Input: part model. Units: mm. Frame: model coordinates. Face numbers are marked on the shaded views. A direction names the side the tool comes from. Give positions to 0.01 mm unless a question says otherwise; leave off trailing zeros. Loops run counter-clockwise (first coordinate to the right, second up) from the corner with the lowest first, then second, coordinate; pieces in that order, holes last. Notation, with made-up numbers: (-1, 73) -> (3, 73) arc R12 cw to (3, 88) -> close; hole circle Ø6 at (30.5, 68). An arc over 180 degrees is marked (long way). Answer in a Markdown table with one row per item. Add a question column.
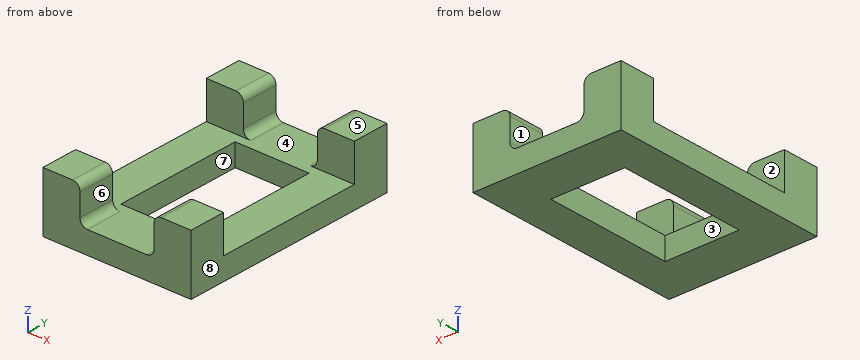
```python
from build123d import *

# Parameters (mm, degrees)
F0_W      = 40
F0_H      = 60
F1_DEPTH  = 6
F2_W      = 10
F2_H      = 10
F3_DEPTH  = 10
F13_R     = 2
F14_W     = 20
F14_H     = 35
F15_DEPTH = 25


# Not quite as in the source:
# - the program builds the solid bodies; features that only make, move or delete a surface that nothing else refers to are left out


with BuildPart() as f1:
    # F0 (on Top) → F1 (new body)
    with BuildSketch(Plane.XY):
        Rectangle(F0_W, F0_H)
    extrude(amount=-F1_DEPTH)

    # F2 (on face) → F3 (join)
    with BuildSketch(Plane.XY):
        with Locations((-15, 25)):
            Rectangle(F2_W, F2_H)
        with Locations((15, 25)):
            Rectangle(F2_W, F2_H)
        with Locations((15, -25)):
            Rectangle(F2_W, F2_H)
        with Locations((-15, -25)):
            Rectangle(F2_W, F2_H)
    extrude(amount=F3_DEPTH)

    # F13
    f13_edges = [f1.edges().sort_by_distance(p)[0] for p in [
        (-10, 25, 10),
        (-10, -25, 10),
        (-10, -25, 0),
        (-10, 25, 0),
        (10, -25, 10),
        (10, 25, 10),
        (10, -25, 0),
        (10, 25, 0),
    ]]
    fillet(f13_edges, radius=F13_R)

    # F14 (on face) → F15 (cut)
    with BuildSketch(Plane.XY):
        Rectangle(F14_W, F14_H)
    extrude(amount=-F15_DEPTH, mode=Mode.SUBTRACT)


solid = f1.part
```
1) Pull-direction query (X, two-part tool) for the marked faces 5, 6, 7 and 8; classes: +X half, -X half, draft (parallel to the pull), parting line (faces both ways), or undercut.
2) Pin query (flat end, axial travel): pin 1 (5 mm diameter, centred on y = -13.5, z = 4.5, fed in from -X). Return the tip coordinate at first contact, or that it passes through.
3) Section C-C on x = 3.5. Output: boundary loops of the cut face in (y, z), and give its area (3 significant figures).
4) Material intervals for line 1 along Y through (x, z) = (14, 5.25); line 2 along X through (y, z) = (22, 6.5); line 3 along Y through (x, z) = (4, -5), sorted ascending.
5) Section B-B on y = -15. Output: boundary loops of the cut face in (x, z).
6) Section A-A on z = 4. Output: boundary loops of the cut face in (x, y).
7) Reachability of the marked faces 1, 2, 3 and 4 from +Z, -Z, +X, -X, +Y, -Y: full face, straight path, thin tool, end or side. Return the list, or none.
8) Section D-D on z = -4. Output: boundary loops of the cut face in (x, y), and give its area (3 significant figures).
Working result:
| question | item | result |
|---|---|---|
| 1 | face 5 | draft |
| 1 | face 6 | undercut |
| 1 | face 7 | undercut |
| 1 | face 8 | +X half |
| 2 | pin 1 | passes through |
| 3 | outline | (-30, -6) -> (-17.5, -6) -> (-17.5, 0) -> (-30, 0) -> close; (17.5, -6) -> (30, -6) -> (30, 0) -> (17.5, 0) -> close |
| 3 | area | 150 mm2 |
| 4 | line 1 | y = -30 to -20, 20 to 30 |
| 4 | line 2 | x = -20 to -10, 10 to 20 |
| 4 | line 3 | y = -30 to -17.5, 17.5 to 30 |
| 5 | outline | (-20, -6) -> (-10, -6) -> (-10, 0) -> (-20, 0) -> close; (10, -6) -> (20, -6) -> (20, 0) -> (10, 0) -> close |
| 6 | outline | (-20, -30) -> (-10, -30) -> (-10, -20) -> (-20, -20) -> close; (-20, 20) -> (-10, 20) -> (-10, 30) -> (-20, 30) -> close; (10, -30) -> (20, -30) -> (20, -20) -> (10, -20) -> close; (10, 20) -> (20, 20) -> (20, 30) -> (10, 30) -> close |
| 7 | face 1 | +Z, +Y, -Y |
| 7 | face 2 | +Z, +X, -X |
| 7 | face 3 | +Z, -Z |
| 7 | face 4 | +Z |
| 8 | outline | (-20, -30) -> (20, -30) -> (20, 30) -> (-20, 30) -> close; hole (-10, -17.5) -> (10, -17.5) -> (10, 17.5) -> (-10, 17.5) -> close |
| 8 | area | 1,700 mm2 |
